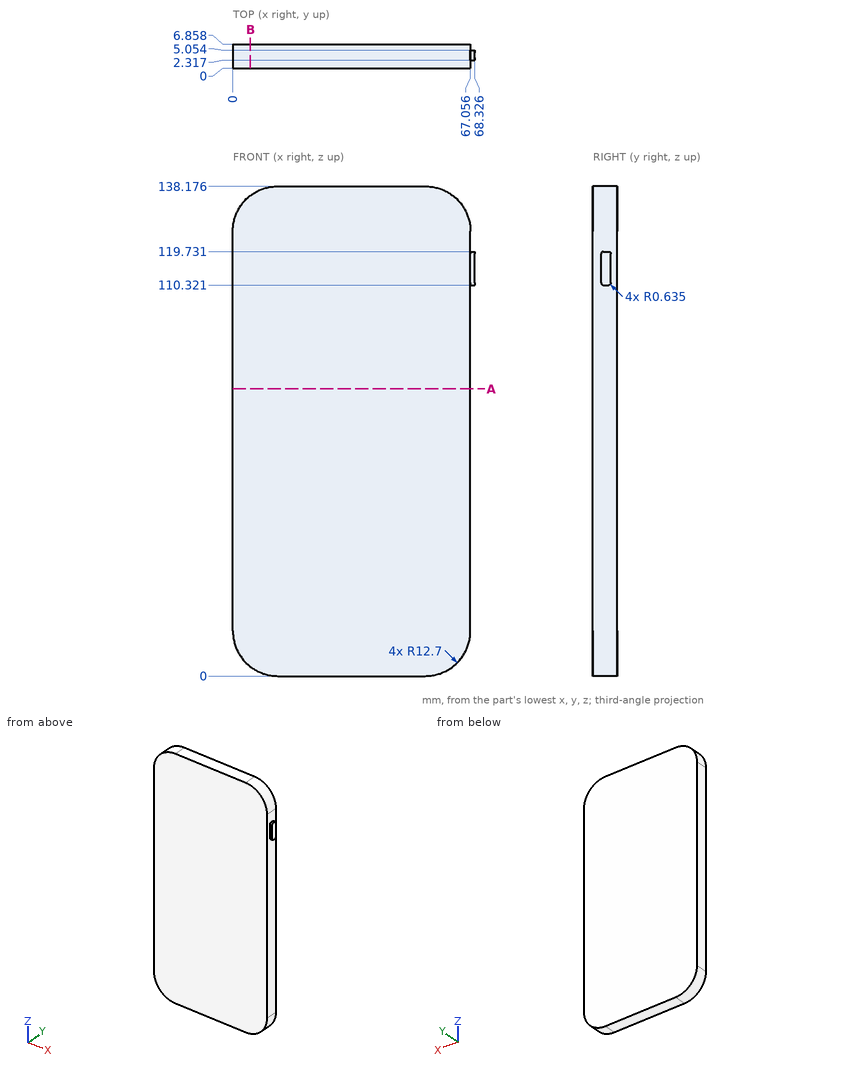
Job drawing, mm, ordinate dimensions from the low corner. One solid piece. Round coordinates to 2 decimals unless told otherwise and drop trailing zeros. Order: outer loops, then holes, each group sorted by start corner. A loop starts at its lowest first (then second) coordinate and runs counter-clockwise, first axis right, second up. Notation, with made-up numbers: M 44.25,49.5 L 89.25,49.5 A10 cw 89.25,59.5 Z; hole C 87.5,81.25 d1. An arc over 180 degrees is marked long. Write each question's results on one line, items separated by ' | '. Start each with the question number.
(1) Drop flat-ended pins along their axis: pin 1 (3 mm diameter, centred on y = 2, z = 93.5, fed in from -X); pin 2 (1 mm diameter, centred on y = 5, z = 70, fed in from +X); pin 3 (1.4 mm diameter, centred on x = 68, y = 3.5, fed in from +Z). Give the stop position or say it passes through.
(2) Saw through at B-B, the plane x = 5. Give the cut face in (y, z) (1 decimal).
(3) Probe probe 1 along X at (y, z) = (4, 78); probe 2 along Z at (x, y) = (12, 4.75); probe 3 along Z at (x, y) = (64, 5) (1 decimal). List the from-to ranges inside material, lowest first. Write a range as from..to.
(4) Saw through at A-A, the plane z = 81. Give the cut face in (x, y).
Established:
1) pin 1: stops at x = 0 | pin 2: stops at x = 67.06 | pin 3: stops at z = 119.73
2) outline: M 0,2.6 L 6.9,2.6 L 6.9,135.6 L 0,135.6 Z
3) probe 1: x = 0..67.06 | probe 2: z = 0.02..138.16 | probe 3: z = 4.4..133.7
4) outline: M 0,0 L 67.06,0 L 67.06,6.86 L 0,6.86 Z
